Can you work these out from the model? Positions are in its coordinate system, mm. Coordinates: 2 decimals unless noted, no trailing zeros. Loops run counter-clockwise (first coordinate to the right, second up) from the corner with the lowest first, then second, coordinate; pieces in that order, holes last. Notation, with made-up numbers: (-36, -10) -> (-28, -10) arc R31 ccw to (-28, 26) -> close; hole circle Ø4 at (65, -18). An arc over 180 degrees is marked (long way). Put each result on its own line as item: value. Start each with the question number.
Item 1: Please list where these lines run through material, in increasing order: L1, parallel to X at y = 1.25, z = -3; L2, parallel to Z at x = 8, y = 3.5; L3, parallel to X at y = 2, z = -40. Write a range as from..to.
Item 2: Will these pins go through, and if not, where does the flat tip stop? P1, Ø3.5, axis at x = 0, y = 6.5, coming from the -Z side; P2, Ø5, axis at x = -13.967, z = 37.5, coming from the -Y side; P3, Ø1, axis at y = 1, z = -14, coming from the +X side; P4, Ø1.5, axis at y = -1, z = -36, coming from the +X side.
Item 3: If we section it at D-D on x = -13: Please give me the cut outline in (y, z).
Item 4: If we section it at C-C on z = 37.5: Please give me the cut outline in (x, y), plus the area to 3 significant figures.
Item 5: If we section it at B-B on y = -1.5: Please give me the cut outline in (x, z), plus the area to 3 significant figures.
Item 6: If we section it at A-A on x = -22.5: Please give me the cut outline in (y, z), plus the area to 3 significant figures.
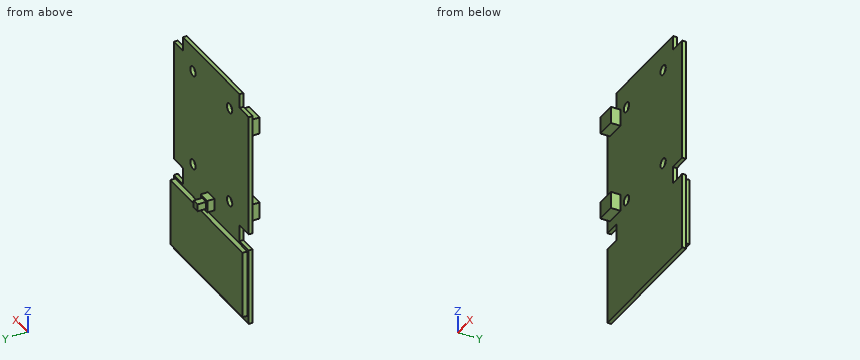
Autodesk Inventor part; units mm, degrees
ref_plane "YZ Plane" through (0, 0, 0) normal (1, 0, 0) x (0, 1, 0)
ref_plane "XZ Plane" through (0, 0, 0) normal (0, 1, 0) x (-1, 0, 0)
ref_plane "XY Plane" through (0, 0, 0) normal (0, 0, 1) x (1, 0, 0)
sketch "Sketch1" plane through (0, 0, 0) normal (0, 1, 0) x (-1, 0, 0)
  line L0 (-28.5, -48) -> (28.5, -48)
  line L1 (28.5, 48) -> (-28.5, -48) construction
  line L2 (-28.5, 48) -> (28.5, -48) construction
  line L3 (-28.5, -48) -> (-28.5, -16)
  line L4 (-28.5, -16) -> (-21.5, -16)
  line L5 (-21.5, -16) -> (-21.5, -9)
  line L6 (-21.5, -9) -> (-28.5, -9)
  line L7 (0, -48) -> (0, 48)
  line L8 (21.5, -16) -> (21.5, -9)
  line L9 (28.5, -16) -> (21.5, -16)
  line L10 (21.5, -9) -> (28.5, -9)
  line L11 (-28.5, -9) -> (-28.5, 16.5)
  line L12 (-28.5, 16.5) -> (28.5, 16.5)
  line L13 (21.5, 42) -> (28.5, 42)
  line L14 (-28.5, -48) -> (-13.5, -48)
  line L15 (-13.5, -48) -> (-13.5, -3)
  line L16 (28.5, 42) -> (28.5, -9)
  line L17 (28.5, -16) -> (28.5, -48)
  line L18 (-28.5, 16.5) -> (-28.5, 42)
  line L19 (-28.5, -3) -> (-13.967, -3)
  circle A0 centre (-13.967, -3) radius 2
  line L20 (-28.5, 37) -> (-13.967, 37)
  circle A1 centre (13.967, -3) radius 2
  line L21 (21.5, 48) -> (21.5, 42)
  line L22 (-28.5, 42) -> (-21.5, 42)
  line L23 (-21.5, 42) -> (-21.5, 48)
  line L24 (-21.5, 48) -> (21.5, 48)
  line L25 (-13.967, 48) -> (-13.967, 37.5)
  line L26 (-13.967, 48) -> (-3.467, 48) construction
  line L27 (13.967, 48) -> (13.967, 37.5)
  circle A2 centre (13.967, 37.5) radius 2
  circle A3 centre (-13.967, 37.5) radius 2
  point P0 (0, 0)
  dimension "d0" = 57
  dimension "d1" = 96
  dimension "d2" = 32
  dimension "d3" = 7
  dimension "d4" = 7
  dimension "d5" = 25.5
  dimension "d7" = 45
  dimension "d40" = 14.533
  dimension "d41" = 4
  dimension "d42" = 14.533
  dimension "d50" = 14.533
  dimension "d57" = 7
  dimension "d59" = 10.5
  dimension "d60" = 90
  dimension "d61" = 10.5
  dimension "d62" = 4
  dimension "d63" = 4
extrude "Extrusion2" add sketch "Sketch1" along normal blind 1.6 contours L3 L4 L5 L6 L11 L19 A0 L15 L0 | L15 A0 L19 L11 L12 L7 L0 | L7 L12 L16 L10 L8 L9 L17 L0 | A0 | L12 L18 L20 A3 L25 L24 L7 | A2 | L7 L24 L21 L13 L16 L12 | L25 A3 L20 L18 L22 L23 L24 | A3 | A1
sketch "Sketch3" plane through (0, 1.6, 0) normal (0, 1, 0) x (1, 0, 0)
  line L0 (28.5, 48) -> (-28.5, 48)
  line L1 (28.5, 48) -> (27.5, 48)
  line L2 (27.5, 48) -> (27.5, 45)
  line L3 (27.5, 45) -> (28.5, 45)
  line L4 (28.5, 45) -> (28.5, 48)
  line L5 (27.5, 45) -> (-27.5, 45)
  line L6 (-27.5, 45) -> (-27.5, 17)
  line L7 (-27.5, 17) -> (27.5, 17)
  line L8 (27.5, 17) -> (27.5, 45)
  point P0 (0, 0)
  dimension "d16" = 1
  dimension "d17" = 3
  dimension "d18" = 55
  dimension "d19" = 28
extrude "Extrusion3" add sketch "Sketch3" along normal blind 2 contours L8 L7 L6 L5
sketch "Sketch4" plane through (0, 1.6, 0) normal (0, 1, 0) x (1, 0, 0)
  line L0 (-2.5, 8.5) -> (2.5, 8.5)
  line L1 (2.5, 8.5) -> (2.5, 13.5)
  line L2 (2.5, 13.5) -> (-2.5, 13.5)
  line L3 (-2.5, 13.5) -> (-2.5, 8.5)
  line L4 (-2.5, 8.5) -> (2.5, 13.5) construction
  line L5 (2.5, 8.5) -> (-2.5, 13.5) construction
  point P0 (0, 0)
  point P1 (-21.5, -46.725)
  point P2 (21.5, -46.725)
extrude "Extrusion4" add sketch "Sketch4" along normal blind 3
sketch "Sketch5" plane through (0, 4.6, 0) normal (0, 1, 0) x (1, 0, 0)
  line L0 (-2.5, 8.5) -> (-2.5, 13.5)
  line L1 (-2.5, 13.5) -> (0, 13.5)
  line L2 (0, 13.5) -> (0, 11)
  line L3 (0, 11) -> (-2.5, 11)
  line L4 (-2.5, 11) -> (-2.5, 13.5)
  line L5 (-5, 6) -> (5, 6)
  line L6 (5, 6) -> (5, 16)
  line L7 (5, 16) -> (-5, 16)
  line L8 (-5, 16) -> (-5, 6)
  line L9 (-5, 6) -> (5, 16) construction
  line L10 (5, 6) -> (-5, 16) construction
  point P0 (0, 0)
  dimension "d64" = 10
  dimension "d65" = 10
sketch "Sketch6" plane through (0, 4.6, 0) normal (0, 1, 0) x (1, 0, 0)
  line L0 (2.5, 8.5) -> (2.5, 13.5)
  line L1 (2.5, 13.5) -> (0, 13.5)
  line L2 (0, 13.5) -> (0, 11)
  line L3 (0, 11) -> (2.5, 11)
  line L4 (2.5, 11) -> (2.5, 13.5)
  line L5 (-1.5, 9.5) -> (1.5, 9.5)
  line L6 (1.5, 9.5) -> (1.5, 12.5)
  line L7 (1.5, 12.5) -> (-1.5, 12.5)
  line L8 (-1.5, 12.5) -> (-1.5, 9.5)
  line L9 (-1.5, 9.5) -> (1.5, 12.5) construction
  line L10 (1.5, 9.5) -> (-1.5, 12.5) construction
  point P0 (0, 0)
  dimension "d29" = 3
  dimension "d30" = 3
extrude "Extrusion5" add sketch "Sketch6" along normal blind 3.5 contours L6 L5 L8 L7 L2 L3 | L3 L2 L7 L6
sketch "Sketch7" plane through (0, 0, 0) normal (0, -1, 0) x (1, 0, 0)
  line L0 (28.5, -48) -> (-28.5, -48)
  line L1 (-28.5, -48) -> (-26.5, -48)
  line L2 (-26.5, -48) -> (-26.5, -5)
  line L3 (-26.5, -5) -> (-28.5, -5)
  line L4 (-28.5, -5) -> (-28.5, -48)
  line L5 (-26.5, -5) -> (-18.5, -5)
  line L6 (-18.5, -5) -> (-18.5, 2)
  line L7 (-18.5, 2) -> (-26.5, 2)
  line L8 (-26.5, 2) -> (-26.5, -5)
  line L9 (-26.5, 2) -> (-26.5, 17)
  line L10 (-26.5, 17) -> (0, 17)
  line L11 (-18.5, 32) -> (-26.5, 32)
  line L12 (-18.5, 39) -> (-18.5, 32)
  line L13 (-26.5, 39) -> (-18.5, 39)
  line L14 (-26.5, 32) -> (-26.5, 39)
  point P0 (0, 0)
  dimension "d33" = 2
  dimension "d34" = 43
  dimension "d35" = 8
  dimension "d36" = 7
  dimension "d37" = 15
extrude "Extrusion6" add sketch "Sketch7" along normal blind 4 contours L8 L7 L6 L5 | L11 L14 L13 L12
extrude "Extrusion7" cut sketch "Sketch1" along normal blind 10 contours A0
extrude "Extrusion8" cut sketch "Sketch1" along normal blind 10 contours A1
extrude "Extrusion9" cut sketch "Sketch1" along normal blind 10 contours A2 | A3
properties part number "Cheapstat"
Solutions:
1. L1: -28.5..-15.97, -11.97..11.97, 15.97..28.5
1. L2: -45..-17
1. L3: -27.5..27.5
2. P1: z = -12.5
2. P2: y = 0
2. P3: x = 21.5
2. P4: through
3. outline: (0, -48) -> (1.6, -48) -> (1.6, -45) -> (3.6, -45) -> (3.6, -17) -> (1.6, -17) -> (1.6, -4.75) -> (0, -4.75) -> close; (0, -1.25) -> (1.6, -1.25) -> (1.6, 35.75) -> (0, 35.75) -> close; (0, 39.25) -> (1.6, 39.25) -> (1.6, 48) -> (0, 48) -> close
4. outline: (-28.5, 0) -> (-26.5, 0) -> (-26.5, -4) -> (-18.5, -4) -> (-18.5, 0) -> (-15.97, 0) -> (-15.97, 1.6) -> (-28.5, 1.6) -> close; (-11.97, 0) -> (11.97, 0) -> (11.97, 1.6) -> (-11.97, 1.6) -> close; (15.97, 0) -> (28.5, 0) -> (28.5, 1.6) -> (15.97, 1.6) -> close
4. area: 110 mm^2
5. outline: (-26.5, -5) -> (-18.5, -5) -> (-18.5, 2) -> (-26.5, 2) -> close; (-26.5, 32) -> (-18.5, 32) -> (-18.5, 39) -> (-26.5, 39) -> close
5. area: 112 mm^2
6. outline: (-4, -5) -> (0, -5) -> (0, -9) -> (1.6, -9) -> (1.6, 42) -> (0, 42) -> (0, 39) -> (-4, 39) -> (-4, 32) -> (0, 32) -> (0, 2) -> (-4, 2) -> close; (0, -48) -> (1.6, -48) -> (1.6, -45) -> (3.6, -45) -> (3.6, -17) -> (1.6, -17) -> (1.6, -16) -> (0, -16) -> close
6. area: 245 mm^2
